Work out the finished part from the listing and answer in its coordinate system (mm). Coordinates: 2 decimals unless noted, no trailing zeros. Order: outer loops, then holes, each group sorted by start corner. A loop starts at its lowest first (then second) coordinate and runs counter-clockwise, first axis right, second up. Notation, with made-up numbers: (-32, 34) -> (4, 34) arc R24 ccw to (4, 68) -> close; hole circle Ø2 at (48, 65). An arc over 180 degrees is marked (long way). Use one line per item in the form item = value.
from build123d import *

# Parameters (mm, degrees)
SKETCH4_R           = 2
BOSS_EXTRUDE3_DEPTH = 6
SKETCH6_R           = 3.276903459
BOSS_EXTRUDE4_DEPTH = 6
CUT_EXTRUDE1_DEPTH  = 10


with BuildPart() as part:
    # Sketch4 → Boss-Extrude3 (new body)
    with BuildSketch(Plane.XY):
        with BuildLine():
            ThreePointArc((11.330682707, 3.9516616), (8.917819898, 4.428819506), (6.681915604, 3.403968986))
            ThreePointArc((6.681915604, 3.403968986), (6.066818441, 4.407801607), (5.302192362, 5.302995112))
            ThreePointArc((5.302192362, 5.302995112), (6.967815552, 7.112770233), (7.259627029, 9.554989032))
            ThreePointArc((7.259627029, 9.554989032), (7.053423028, 9.708203932), (6.843986457, 9.856969584))
            ThreePointArc((6.843986457, 9.856969584), (4.61147306, 8.824753264), (3.40498051, 6.681400208))
            ThreePointArc((3.40498051, 6.681400208), (2.317318441, 7.131972816), (1.172541409, 7.406763642))
            ThreePointArc((1.172541409, 7.406763642), (1.456299749, 9.849931218), (0.256880001, 11.997250213))
            ThreePointArc((0.256880001, 11.997250213), (0, 12), (-0.256880001, 11.997250213))
            ThreePointArc((-0.256880001, 11.997250213), (-1.456299749, 9.849931218), (-1.172541409, 7.406763642))
            ThreePointArc((-1.172541409, 7.406763642), (-2.317318441, 7.131972816), (-3.404980509, 6.681400207))
            ThreePointArc((-3.404980509, 6.681400207), (-4.61147306, 8.824753264), (-6.843986457, 9.856969584))
            ThreePointArc((-6.843986457, 9.856969584), (-7.053423028, 9.708203933), (-7.259627029, 9.554989032))
            ThreePointArc((-7.259627029, 9.554989032), (-6.967815552, 7.112770233), (-5.302192362, 5.302995112))
            ThreePointArc((-5.302192362, 5.302995112), (-6.066818441, 4.407801607), (-6.681915604, 3.403968986))
            ThreePointArc((-6.681915604, 3.403968986), (-8.917819898, 4.428819506), (-11.330682707, 3.9516616))
            ThreePointArc((-11.330682707, 3.9516616), (-11.412678196, 3.708203933), (-11.489443278, 3.463046803))
            ThreePointArc((-11.489443278, 3.463046803), (-9.817862641, 1.658772773), (-7.406586048, 1.173662691))
            ThreePointArc((-7.406586048, 1.173662691), (-7.499, 0), (-7.406586048, -1.173662691))
            ThreePointArc((-7.406586048, -1.173662691), (-9.817862641, -1.658772773), (-11.489443278, -3.463046803))
            ThreePointArc((-11.489443278, -3.463046803), (-11.412678196, -3.708203933), (-11.330682707, -3.9516616))
            ThreePointArc((-11.330682707, -3.9516616), (-8.917819898, -4.428819506), (-6.681915604, -3.403968986))
            ThreePointArc((-6.681915604, -3.403968986), (-6.066818441, -4.407801607), (-5.302192362, -5.302995112))
            ThreePointArc((-5.302192362, -5.302995112), (-6.967815552, -7.112770233), (-7.259627029, -9.554989032))
            ThreePointArc((-7.259627029, -9.554989032), (-7.053423028, -9.708203932), (-6.843986457, -9.856969584))
            ThreePointArc((-6.843986457, -9.856969584), (-4.61147306, -8.824753264), (-3.404980509, -6.681400207))
            ThreePointArc((-3.404980509, -6.681400207), (-2.317318441, -7.131972816), (-1.172541409, -7.406763642))
            ThreePointArc((-1.172541409, -7.406763642), (-1.456299749, -9.849931218), (-0.256880001, -11.997250213))
            ThreePointArc((-0.256880001, -11.997250213), (0, -12), (0.256880001, -11.997250213))
            ThreePointArc((0.256880001, -11.997250213), (1.456299749, -9.849931218), (1.172541409, -7.406763642))
            ThreePointArc((1.172541409, -7.406763642), (2.317318441, -7.131972816), (3.404980509, -6.681400207))
            ThreePointArc((3.404980509, -6.681400207), (4.61147306, -8.824753264), (6.843986457, -9.856969584))
            ThreePointArc((6.843986457, -9.856969584), (7.053423027, -9.708203933), (7.259627029, -9.554989032))
            ThreePointArc((7.259627029, -9.554989032), (6.967815552, -7.112770233), (5.302192362, -5.302995112))
            ThreePointArc((5.302192362, -5.302995112), (6.066818441, -4.407801607), (6.681915604, -3.403968986))
            ThreePointArc((6.681915604, -3.403968986), (8.917819898, -4.428819506), (11.330682707, -3.9516616))
            ThreePointArc((11.330682707, -3.9516616), (11.412678196, -3.708203932), (11.489443278, -3.463046803))
            ThreePointArc((11.489443278, -3.463046803), (9.817862641, -1.658772773), (7.406586048, -1.173662691))
            ThreePointArc((7.406586048, -1.173662691), (7.499, 0), (7.406586048, 1.173662691))
            ThreePointArc((7.406586048, 1.173662691), (9.817862641, 1.658772773), (11.489443278, 3.463046803))
            ThreePointArc((11.489443278, 3.463046803), (11.412678196, 3.708203932), (11.330682707, 3.9516616))
        make_face()
        Circle(SKETCH4_R, mode=Mode.SUBTRACT)
    extrude(amount=BOSS_EXTRUDE3_DEPTH)

    # Sketch6 → Boss-Extrude4 (add)
    with BuildSketch(Plane.XY.offset(6)):
        Circle(SKETCH6_R)
    extrude(amount=-BOSS_EXTRUDE4_DEPTH)

    # Sketch7 → Cut-Extrude1 (cut)
    with BuildSketch(Plane.XY.offset(6)):
        with BuildLine():
            Line((-1.792651667, 1.67), (1.792651667, 1.67))
            ThreePointArc((1.792651667, 1.67), (0, -2.45), (-1.792651667, 1.67))
        make_face()
    extrude(amount=-CUT_EXTRUDE1_DEPTH, mode=Mode.SUBTRACT)


solid = part.part
(1) Section A-A on y = 0 is taken. Write down the section's boundary in (x, z).
Data:
outline = (-7.5, 0) -> (-2.45, 0) -> (-2.45, 6) -> (-7.5, 6) -> close; (2.45, 0) -> (7.5, 0) -> (7.5, 6) -> (2.45, 6) -> close
(2) The mould has two halves that part along Y. Classify faces 1 (the cylindrical face through (-9.848, 1.676, 2.958)), 2 (the flat face through (-3, 0, 6)): released by +Y, released by -Y, zero draft, split by the parting line, or undercut.
Data:
face_1 = undercut
face_2 = zero draft
(3) Section C-C on x = -9.5 is taken. Write down the section's boundary in (y, z), plus the area to 3 significant figures.
Data:
outline = (-4.45, 0) -> (-1.5, 0) -> (-1.5, 6) -> (-4.45, 6) -> close; (1.5, 0) -> (4.45, 0) -> (4.45, 6) -> (1.5, 6) -> close
area = 35.5 mm²
(4) Section B-B on y = -8.5 is taken. Write down the section's boundary in (x, z).
Data:
outline = (-7.32, 0) -> (-4.3, 0) -> (-4.3, 6) -> (-7.32, 6) -> close; (-1.49, 0) -> (1.49, 0) -> (1.49, 6) -> (-1.49, 6) -> close; (4.3, 0) -> (7.32, 0) -> (7.32, 6) -> (4.3, 6) -> close
(5) Straight lines are drawn through the part: line 1 along X through (y, z) = (0, 4.75); line 2 along Y through (x, z) = (-6.5, 3.5); line 3 along X through (y, z) = (9, 0.75). For each, find the intervals that lie inside material, in ascending order.
Data:
line_1 = -7.5 to -2.45, 2.45 to 7.5
line_2 = -9.8 to -6.34, -3.74 to 3.74, 6.34 to 9.8
line_3 = -7.33 to -4.81, -1.53 to 1.53, 4.81 to 7.33
(6) Section D-D on x = -5.75 is taken. Write down the section's boundary in (y, z), plus the area to 3 significant figures.
Data:
outline = (-9.56, 0) -> (-5.6, 0) -> (-5.6, 6) -> (-9.56, 6) -> close; (-4.81, 0) -> (4.81, 0) -> (4.81, 6) -> (-4.81, 6) -> close; (5.6, 0) -> (9.56, 0) -> (9.56, 6) -> (5.6, 6) -> close
area = 105 mm²
